For this review, take the finished solid that the model builds, in its own axes (mm). Round coordinates to 2 decimals unless told otherwise and drop trailing zeros. Write each loop counter-clockwise with the first axis right and the second up, starting at its lowest first coordinate (ties: lowest second). Pieces come first, ordered by that corner, then holes. Notation, with made-up numbers: M 83,67.5 L 122,67.5 A34 cw 122,103.5 Z; hole C -38,35 d5. An arc over 180 degrees is marked long. Answer in a Markdown table with one row per item.
Autodesk Inventor part; units mm, degrees
ref_plane "YZ Plane" through (0, 0, 0) normal (1, 0, 0) x (0, 1, 0)
ref_plane "XZ Plane" through (0, 0, 0) normal (0, 1, 0) x (-1, 0, 0)
ref_plane "XY Plane" through (0, 0, 0) normal (0, 0, 1) x (1, 0, 0)
sketch "Sketch1" plane through (0, 0, 0) normal (0, 1, 0) x (-1, 0, 0)
  circle A0 centre (0, 0) radius 17.78
  dimension "d0" = 35.56
extrude "Extrusion1" add sketch "Sketch1" along normal blind 1.27
sketch "Sketch2" plane through (0, 1.27, 0) normal (0, 1, 0) x (1, 0, 0)
  circle A0 centre (0, 0) radius 17.78
hole "Hole1" at (0, 1.27, 0) direction (0, -1, 0) diameter 6.35 end through all
sketch "Sketch3" plane through (0, 1.27, 0) normal (0, 1, 0) x (1, 0, 0)
  line L0 (0, 0) -> (-13.6144, 0)
  dimension "d10" = 13.6144
hole "Hole2" at (-13.6144, 1.27, 0) direction (0, -1, 0) diameter 4.9022 end through all
pattern_circular "Circular Pattern1" count 3 over 360 about axis through (0, -49.0355, 0) along (0, 1, 0) of "Hole2"
sketch "Sketch5" plane through (0, 1.27, 0) normal (0, 1, 0) x (1, 0, 0)
  circle A0 centre (-13.6144, 0) radius 2.4511
  circle A1 centre (6.8072, 11.7904) radius 2.4511
  line L0 (-13.6144, 0) -> (6.8072, 11.7904)
  circle A2 centre (6.8072, -11.7904) radius 2.4511
  line L1 (6.8072, 11.7904) -> (6.8072, -11.7904)
  line L2 (6.8072, -11.7904) -> (-13.6144, 0)
  line L3 (-13.6144, 0) -> (-13.6144, -11.7904)
  line L4 (-13.6144, -11.7904) -> (6.8072, -11.7904)
  line L5 (-13.6144, 0) -> (-13.6144, 11.7904)
  line L6 (-13.6144, 11.7904) -> (6.8072, 11.7904)
  circle A3 centre (-3.4036, 11.7904) radius 0.635
  circle A4 centre (-3.4036, -11.7904) radius 0.635
  point P0 (0, 0)
  dimension "d28" = 1.27
hole "Hole4" at (-3.4036, 1.27, 11.7904) at (-3.4036, 1.27, -11.7904) direction (0, -1, 0) diameter 1.905 depth 6.35 tip angle 118
properties part number "buffer" material "PBT Plastic"
Q1. Take a section at D-D (x = 8). State the section outline as (y, z) points, then the cut area to 3 significant figures.
Found:
| item | result |
|---|---|
| outline | M 0,-15.88 L 1.27,-15.88 L 1.27,-13.93 L 0,-13.93 Z; M 0,-9.65 L 1.27,-9.65 L 1.27,9.65 L 0,9.65 Z; M 0,13.93 L 1.27,13.93 L 1.27,15.88 L 0,15.88 Z |
| area | 29.5 mm² |
Q2. Mouldability with a two-part tool opening along X and no side actions: class faces 1 (the face through (4.377, 0.626, -12.11)), 2 (the face through (3.85, 0.63, 17.36)), 3 (the face through (0, 1.27, -4)) as +X half, -X half, draft (parallel to the pull), parting line (faces both ways), or undercut.
Found:
| item | result |
|---|---|
| face 1 | undercut |
| face 2 | parting line |
| face 3 | draft |
Q3. Take a section at A-A (z = 0). State the section outline as (x, y) points (1 decimal).
Found:
| item | result |
|---|---|
| outline | M -17.8,0 L -16.1,0 L -16.1,1.3 L -17.8,1.3 Z; M -11.2,0 L -3.2,0 L -3.2,1.3 L -11.2,1.3 Z; M 3.2,0 L 17.8,0 L 17.8,1.3 L 3.2,1.3 Z |
Q4. Take a section at B-B (x = 0). State the section outline as (y, z) points (3 decimals), then the cut area to 3 significant figures.
Found:
| item | result |
|---|---|
| outline | M 0,-17.78 L 1.27,-17.78 L 1.27,-3.175 L 0,-3.175 Z; M 0,3.175 L 1.27,3.175 L 1.27,17.78 L 0,17.78 Z |
| area | 37.1 mm² |
Q5. Take a section at C-C (y = 1.05). State how many separate pieces and enclosed holes the cut face has, then the cut area to 3 significant figures.
Found:
| item | result |
|---|---|
| separate pieces | 1 |
| enclosed holes | 6 |
| area | 899 mm² |
Q6. Insertion check: P1, Ø4, axis at x = 6.81, z = -11.79, coming from the -Y side. The pin has a flat end and moves straight along its axis. Give the tip position at first contact, or say it passes through.
Found:
| item | result |
|---|---|
| P1 | through |
Q7. For probe 1 along Z at (x, y) = (6.5, 0.6); probe 2 along Z at (x, y) = (0, 0.45) (3 decimals); probe 3 along X at (y, z) = (1, -0.5), list the stretches that pass through material, from the lowest coordinate up.
Found:
| item | result |
|---|---|
| probe 1 | -16.55 to -14.22, -9.36 to 9.36, 14.22 to 16.55 |
| probe 2 | -17.78 to -3.175, 3.175 to 17.78 |
| probe 3 | -17.77 to -16.01, -11.21 to -3.14, 3.14 to 17.77 |
